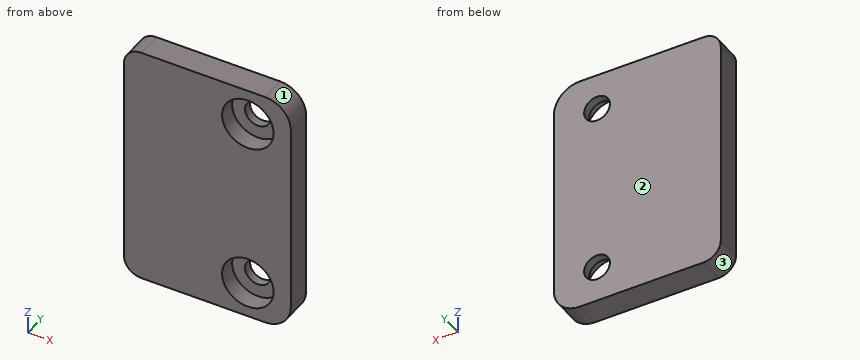
```python
from build123d import *

# Parameters (mm, degrees)
SKETCH1_W           = 19.4
SKETCH1_H           = 28.4
BOSS_EXTRUDE1_DEPTH = 3
FILLET1_R           = 3
FILLET2_R           = 2
SKETCH2_R           = 1.5
CUT_EXTRUDE1_DEPTH  = 4
SKETCH4_R           = 3
CUT_EXTRUDE2_DEPTH  = 2


with BuildPart() as part:
    # Sketch1 → Boss-Extrude1 (new body)
    with BuildSketch(Plane(origin=(0, 0, 0), x_dir=(1, 0, 0), z_dir=(0, 1, 0))):
        Rectangle(SKETCH1_W, SKETCH1_H)
    extrude(amount=BOSS_EXTRUDE1_DEPTH)

    # Fillet1
    fillet1_edges = [part.edges().sort_by_distance(p)[0] for p in [
        (9.7, 1.5, -14.2),
        (9.7, 1.5, 14.2),
    ]]
    fillet(fillet1_edges, radius=FILLET1_R)

    # Fillet2
    fillet2_edges = [part.edges().sort_by_distance(p)[0] for p in [
        (-9.7, 1.5, -14.2),
        (-9.7, 1.5, 14.2),
    ]]
    fillet(fillet2_edges, radius=FILLET2_R)

    # Sketch2 → Cut-Extrude1 (cut, through all)
    with BuildSketch(Plane(origin=(0, 3, 0), x_dir=(1, 0, 0), z_dir=(0, 1, 0))):
        with Locations((4.7, 10)):
            Circle(SKETCH2_R)
        with Locations((4.7, -10)):
            Circle(SKETCH2_R)
    extrude(amount=-CUT_EXTRUDE1_DEPTH, mode=Mode.SUBTRACT)

    # Sketch4 → Cut-Extrude2 (cut)
    with BuildSketch(Plane.XZ):
        with Locations((4.7, 10)):
            Circle(SKETCH4_R)
        with Locations((4.7, -10)):
            Circle(SKETCH4_R)
    extrude(amount=-CUT_EXTRUDE2_DEPTH, mode=Mode.SUBTRACT)


solid = part.part
```
Part model, mm, in its own coordinate system. Face numbers are marked on the shaded views. Coordinates: 2 decimals unless noted, no trailing zeros. Write each loop counter-clockwise with the first axis right and the second up, starting at its lowest first coordinate (ties: lowest second). Pieces come first, ordered by that corner, then holes.
Item 1: Probe line 1 (Z direction, x = 4.7, y = 1); line 2 (Z direction, x = 4.7, y = 2.3); line 3 (X direction, y = 2.6, z = 10). List the from-to ranges inside material, lowest first.
Item 2: Slice it at C-C (y = 2.65). Write the cut outline in (x, z).
Item 3: Mould opens along Z. For the marked faces 1, 2 and 3 say: released by +Z, released by -Z, zero draft, split by the parting line, or undercut.
Item 4: Slice it at D-D (y = 1.15). Write the cut outline in (x, z), and give its area (3 significant figures).
Item 5: Pin check, flat tips, straight feed: pin 1 (2.5 mm diameter, centred on x = 4.7, z = 10, fed in from -Y); pin 2 (3 mm diameter, centred on x = 5.5, z = 10.5, fed in from -Y). Stop position of each tip, or through.
Item 6: Slice it at A-A (z = 10). Write the cut outline in (x, y), and give its area (3 significant figures).
Item 7: Slice it at B-B (x = 4.7). Write the cut outline in (y, z), and give its area (3 significant figures).
Results found:
1. line 1: z = -14.2 to -13, -7 to 7, 13 to 14.2
1. line 2: z = -14.2 to -11.5, -8.5 to 8.5, 11.5 to 14.2
1. line 3: x = -9.7 to 3.2, 6.2 to 9.7
2. outline: (-9.7, -12.2) arc R2 ccw to (-7.7, -14.2) - (6.7, -14.2) arc R3 ccw to (9.7, -11.2) - (9.7, 11.2) arc R3 ccw to (6.7, 14.2) - (-7.7, 14.2) arc R2 ccw to (-9.7, 12.2) - close; hole circle Ø3 at (4.7, -10); hole circle Ø3 at (4.7, 10)
3. face 1: released by +Z
3. face 2: zero draft
3. face 3: released by -Z
4. outline: (-9.7, -12.2) arc R2 ccw to (-7.7, -14.2) - (6.7, -14.2) arc R3 ccw to (9.7, -11.2) - (9.7, 11.2) arc R3 ccw to (6.7, 14.2) - (-7.7, 14.2) arc R2 ccw to (-9.7, 12.2) - close; hole circle Ø6 at (4.7, -10); hole circle Ø6 at (4.7, 10)
4. area: 489 mm2
5. pin 1: passes through
5. pin 2: stops at y = 2
6. outline: (-9.7, 0) - (1.7, 0) - (1.7, 2) - (3.2, 2) - (3.2, 3) - (-9.7, 3) - close; (6.2, 2) - (7.7, 2) - (7.7, 0) - (9.7, 0) - (9.7, 3) - (6.2, 3) - close
6. area: 43.2 mm2
7. outline: (0, -14.2) - (3, -14.2) - (3, -11.5) - (2, -11.5) - (2, -13) - (0, -13) - close; (0, -7) - (2, -7) - (2, -8.5) - (3, -8.5) - (3, 8.5) - (2, 8.5) - (2, 7) - (0, 7) - close; (0, 13) - (2, 13) - (2, 11.5) - (3, 11.5) - (3, 14.2) - (0, 14.2) - close
7. area: 55.2 mm2
